Autodesk Inventor part; units mm, degrees
ref_plane "YZ Plane" through (0, 0, 0) normal (1, 0, 0) x (0, 1, 0)
ref_plane "XZ Plane" through (0, 0, 0) normal (0, 1, 0) x (-1, 0, 0)
ref_plane "XY Plane" through (0, 0, 0) normal (0, 0, 1) x (1, 0, 0)
sketch "Skizze1" plane through (0, 0, 0) normal (0, 0, 1) x (1, 0, 0)
  line L0 (0, 9.9) -> (0, 0)
  line L1 (0, 0) -> (-17.35, 0)
  line L2 (-17.35, 0) -> (-20.8, 3.45)
  line L3 (-20.8, 3.45) -> (-20.8, 6.45)
  line L4 (-20.8, 6.45) -> (-17.35, 9.9)
  line L5 (-17.35, 9.9) -> (0, 9.9)
  circle A0 centre (-15.9, 4.95) radius 2.85
  circle A1 centre (-4.9, 4.95) radius 2.85
  line L6 (-0.5, 9.4) -> (-0.5, 0.5)
  line L7 (-0.5, 0.5) -> (-17.1429, 0.5)
  line L8 (-17.1429, 0.5) -> (-20.3, 3.6571)
  line L9 (-20.3, 3.6571) -> (-20.3, 6.2429)
  line L10 (-20.3, 6.2429) -> (-17.1429, 9.4)
  line L11 (-17.1429, 9.4) -> (-0.5, 9.4)
  circle A2 centre (-15.9, 4.95) radius 2.25
  circle A3 centre (-4.9, 4.95) radius 2.25
  point P0 (0, 4.95)
  dimension "d2" = 20.8
  dimension "d4" = 45
  dimension "d5" = 9.9
  dimension "d6" = 3
  dimension "d8" = 5.7
  dimension "d9" = 11
  dimension "d11" = 4.9
  dimension "d12" = 0.5
  dimension "d13" = 4.5
extrude "Extrusion1" add sketch "Skizze1" against normal blind 20.7 contours L0 L1 L2 L3 L4 L5 | A0 | A1 | L6 L7 L8 L9 L10 L11 | A2 | A3
extrude "Extrusion2" add sketch "Skizze1" against normal blind 23.5 contours A0 | A1 | A2 | A3
extrude "Extrusion3" cut sketch "Skizze1" against normal blind 15 contours L0 L1 L2 L3 L4 L5 | A2 | A3
equation "\"d11\" = -0.5 * d9 + 0.5 * d2"
properties part number "XT90NE-M" material "PC/ABS-Kunststoff"
Geometry: final body of the model. Coordinates: model frame, mm. A direction names the side the tool comes from. Give positions to 0.01 mm unless a question says otherwise; leave off trailing zeros. Write each loop counter-clockwise with the first axis right and the second up, starting at its lowest first coordinate (ties: lowest second). Pieces come first, ordered by that corner, then holes. Notation, with made-up numbers: (27, -9.5) - (55, -9.5) arc R10 ccw to (55, -1.5) - close; hole circle Ø5 at (59, 33). An arc over 180 degrees is marked (long way). Return JSON: item names as keys, results as strings. Group by question number.
1) Set-up query: faces 5 (the flat face through (-5, 5, -15)), 6 (the flat face through (-18.699, 2.056, -7.395)), 7 (the flat face through (-20.3, 5, -7)). Return all of +Z, -Z, +X, -X, +Y, -Y with unobstructed straight access to the full face (end or side cutting, diameter ignored); none if empty.
2) Line query: line 1 (Y direction, x = -4.9, z = -5.25); line 2 (X direction, y = 4.75, z = -10.5); line 3 (X direction, y = 6.5, z = -1). Output: solid intervals per line, ascending.
3) Section A-A on z = -7.5. Return the cut outline in (x, y).
4) Section B-B on x = -12.75. Return the cut outline in (y, z), plus the area to 3 significant figures.
5) First-contact query: P1, Ø0.8, axis at y = 4.5, z = -7.5, coming from the -X side; P2, Ø3.5, axis at x = -5, y = 4.5, coming from the +Z side; P3, Ø7.5, axis at x = -5.5, z = -11, coming from the -Y side. Flat tips, straight axial feed; report the tip coordinate or a pass-through.
6) Section C-C on y = 4.95. Return the cut outline in (x, z), plus the area to 3 significant figures.
7) Section D-D on z = -18.5. Return the cut outline in (x, y).
8) Mould query, pull axis X, two halves, no side actions, for faces 1 (the flat face through (-0.5, 5, -7)), 2 (the flat face through (-9, 9.9, -18)), 3 (the cylindrical face through (-7.747, 5.075, -22.08)), 4 (the flat face through (-19.1, 8.15, -17.81)). Classes: released by +X, released by -X, zero draft, split by the parting line, or undercut.
Filled in:
{
 "1": {"face 5": "+Z", "face 6": "+Z, -X, -Y", "face 7": "+Z, -X, +Y, -Y"},
 "2": {"line 1": "y = 0.5 to 2.7, 7.2 to 9.4", "line 2": "x = -20.3 to -18.14, -13.66 to -7.14, -2.66 to -0.5", "line 3": "x = -20.04 to -17.53, -14.27 to -6.53, -3.27 to -0.5"},
 "3": {"outline": "(-20.3, 3.66) - (-17.14, 0.5) - (-0.5, 0.5) - (-0.5, 9.4) - (-17.14, 9.4) - (-20.3, 6.24) - close; hole circle Ø4.5 at (-15.9, 4.95); hole circle Ø4.5 at (-4.9, 4.95)"},
 "4": {"outline": "(0, -20.7) - (9.9, -20.7) - (9.9, -15) - (9.4, -15) - (9.4, 0) - (0.5, 0) - (0.5, -15) - (0, -15) - close", "area": "190 mm^2"},
 "5": {"P1": "stops at x = -20.3", "P2": "stops at z = -15", "P3": "stops at y = 0.5"},
 "6": {"outline": "(-20.8, -20.7) - (-18.75, -20.7) - (-18.75, -23.5) - (-13.05, -23.5) - (-13.05, -20.7) - (-7.75, -20.7) - (-7.75, -23.5) - (-2.05, -23.5) - (-2.05, -20.7) - (0, -20.7) - (0, -15) - (-0.5, -15) - (-0.5, 0) - (-2.65, 0) - (-2.65, -15) - (-7.15, -15) - (-7.15, 0) - (-13.65, 0) - (-13.65, -15) - (-18.15, -15) - (-18.15, 0) - (-20.3, 0) - (-20.3, -15) - (-20.8, -15) - close", "area": "312 mm^2"},
 "7": {"outline": "(-20.8, 3.45) - (-17.35, 0) - (0, 0) - (0, 9.9) - (-17.35, 9.9) - (-20.8, 6.45) - close"},
 "8": {"face 1": "released by +X", "face 2": "zero draft", "face 3": "undercut", "face 4": "released by -X"}
}
